Could you check a few things on this model? Use its own coordinates, in mm. Face numbers are marked on the shaded views. A direction names the side the tool comes from. Give positions to 0.01 mm unless a question says otherwise; leave off trailing zeros. Loops run counter-clockwise (first coordinate to the right, second up) from the corner with the lowest first, then second, coordinate; pieces in that order, holes last. Notation, with made-up numbers: (25.25, -7) - (34.25, -7) arc R27 cw to (34.25, 18) - close; hole circle Ø11 at (84.5, 15.5). An arc over 180 degrees is marked (long way). One line per item, written item: value. Start each with the question number.
Q1. I want a section at A-A (z = 629.5). Please give me the cut outline in (x, y).
Q2. If we mould it in two halves opening along X, with no side actions, what happens to the marked faces 3, 4 and 5? For each: released by +X, released by -X, zero draft, split by the parting line, or undercut.
Q3. I'm going to push flat-ended pins straight in: P1, Ø12, axis at x = -307, y = 336.5, coming from the -Z side; P2, Ø4, axis at y = 460, z = 105, coming from the +X side. Where does each tip first touch, or does it pass through?
Q4. I want a section at C-C (x = 77). Please give me the cut outline in (y, z), then the cut area to 3 significant figures.
Q5. I want a section at B-B (y = 88.5). Please give me the cut outline in (x, z).
Q6. For the marked faces 1 and 2, which set-ups out of +Z, -Z, +X, -X, +Y, -Y let a thin tool reach every point of the face, with its end or its side?
Q7. If I drill on line 1 (X direction, y = -504, z = 417); line 2 (Z direction, x = -646, y = -397.5); line 3 (Z direction, x = 647, y = -412), over which ranges is the centre line in solid material (lowest first)? Write a range as from..to.
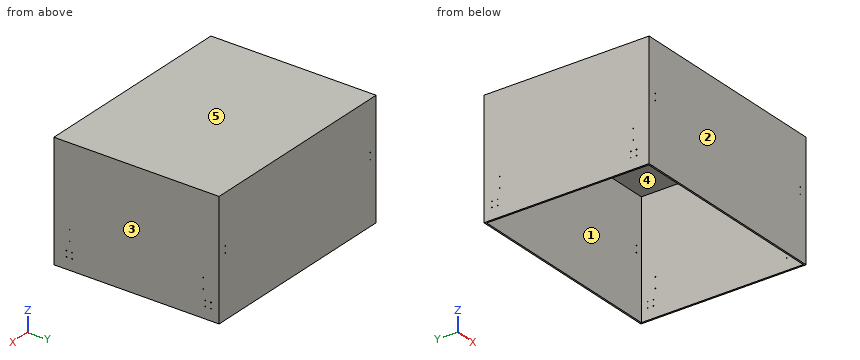
```python
from build123d import *

# Parameters (mm, degrees)
SKETCH1_W               = 1300
SKETCH1_H               = 1020
BOSS_EXTRUDE2_DEPTH     = 720
SKETCH3_W               = 1280
SKETCH3_H               = 1000
CUT_EXTRUDE1_DEPTH      = 710
SKETCH4_R               = 2.5
CUT_EXTRUDE2_DEPTH      = 651
CUT_EXTRUDE2_DEPTH_BACK = 651
SKETCH6_R               = 2.5
CUT_EXTRUDE5_DEPTH      = 3326.5
SKETCH7_R               = 2.5
CUT_EXTRUDE6_DEPTH      = 652
CUT_EXTRUDE6_DEPTH_BACK = 886


with BuildPart() as part:
    # Sketch1 → Boss-Extrude2 (new body)
    with BuildSketch(Plane.XY):
        Rectangle(SKETCH1_W, SKETCH1_H)
    extrude(amount=BOSS_EXTRUDE2_DEPTH)

    # Sketch3 → Cut-Extrude1 (cut)
    with BuildSketch(Plane.XY):
        Rectangle(SKETCH3_W, SKETCH3_H)
    extrude(amount=CUT_EXTRUDE1_DEPTH, mode=Mode.SUBTRACT)

    # Sketch4 → Cut-Extrude2 (cut, two sides)
    with BuildSketch(Plane(origin=(0, 0, 0), x_dir=(0, 0, -1), z_dir=(1, 0, 0))) as cut_extrude2_sk:
        with Locations((-70, 460)):
            Circle(SKETCH4_R)
        with Locations((-105, 460)):
            Circle(SKETCH4_R)
        with Locations((-105, 425)):
            Circle(SKETCH4_R)
        with Locations((-70, 425)):
            Circle(SKETCH4_R)
        with Locations((-105, -432.5)):
            Circle(SKETCH4_R)
        with Locations((-105, -397.5)):
            Circle(SKETCH4_R)
        with Locations((-70, -397.5)):
            Circle(SKETCH4_R)
        with Locations((-70, -432.5)):
            Circle(SKETCH4_R)
    extrude(amount=CUT_EXTRUDE2_DEPTH, mode=Mode.SUBTRACT)
    extrude(cut_extrude2_sk.sketch, amount=-CUT_EXTRUDE2_DEPTH_BACK, mode=Mode.SUBTRACT)

    # Sketch6 → Cut-Extrude5 (cut)
    with BuildSketch(Plane(origin=(650, 0, 0), x_dir=(0, 0, -1), z_dir=(1, 0, 0))):
        with Locations((-105, 460)):
            Circle(SKETCH6_R)
        with Locations((-230, 412.5)):
            Circle(SKETCH6_R)
        with Locations((-165, 412.5)):
            Circle(SKETCH6_R)
        with Locations((-165, -412.5)):
            Circle(SKETCH6_R)
        with Locations((-230, -412.5)):
            Circle(SKETCH6_R)
    extrude(amount=-CUT_EXTRUDE5_DEPTH, mode=Mode.SUBTRACT)

    # Sketch7 → Cut-Extrude6 (cut, two sides)
    with BuildSketch(Plane(origin=(0, 0, 0), x_dir=(1, 0, 0), z_dir=(0, 1, 0))) as cut_extrude6_sk:
        with Locations((600, -417.5)):
            Circle(SKETCH7_R)
        with Locations((600, -377.5)):
            Circle(SKETCH7_R)
        with Locations((-600, -417.5)):
            Circle(SKETCH7_R)
        with Locations((-600, -377.5)):
            Circle(SKETCH7_R)
    extrude(amount=CUT_EXTRUDE6_DEPTH, mode=Mode.SUBTRACT)
    extrude(cut_extrude6_sk.sketch, amount=-CUT_EXTRUDE6_DEPTH_BACK, mode=Mode.SUBTRACT)


solid = part.part
```
Worked answers:
1. outline: (-650, -510) - (650, -510) - (650, 510) - (-650, 510) - close; hole (-640, -500) - (640, -500) - (640, 500) - (-640, 500) - close
2. face 3: released by +X
2. face 4: undercut
2. face 5: zero draft
3. P1: stops at z = 710
3. P2: passes through
4. outline: (-510, 0) - (-500, 0) - (-500, 710) - (500, 710) - (500, 0) - (510, 0) - (510, 720) - (-510, 720) - close
4. area: 24,400 mm²
5. outline: (-650, 0) - (-640, 0) - (-640, 710) - (640, 710) - (640, 0) - (650, 0) - (650, 720) - (-650, 720) - close
6. face 1: -Z
6. face 2: +Z, -Z, +X, -X, -Y
7. line 1: x = -650..-602.45, -597.55..597.55, 602.45..650
7. line 2: z = 0..67.5, 72.5..102.5, 107.5..720
7. line 3: z = 0..162.55, 167.45..227.55, 232.45..720
